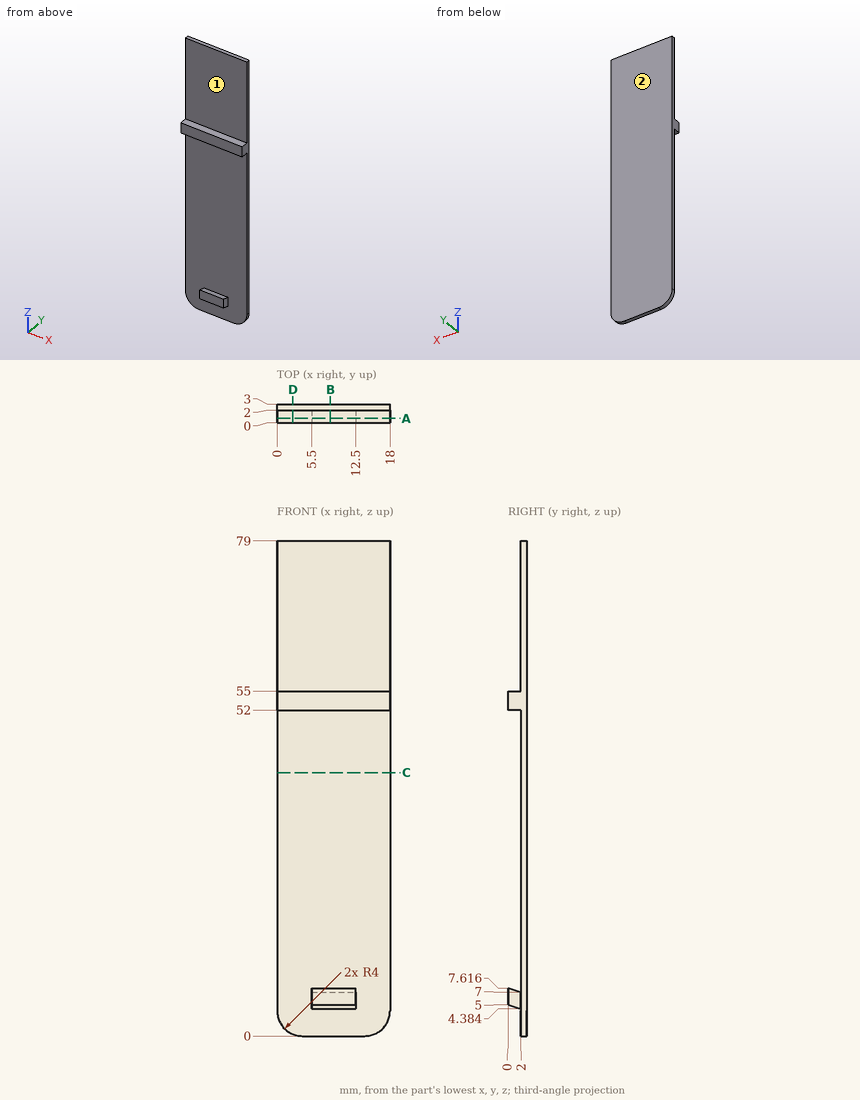
Part print with two shaded views. Sizes in mm from the minimum x, y, z corner. A direction names the side the tool comes from. Round coordinates to 2 decimals unless told otherwise and drop trailing zeros. Order: outer loops, then holes, each group sorted by start corner. A loop starts at its lowest first (then second) coordinate and runs counter-clockwise, first axis right, second up. Notation, with made-up numbers: (7.25, 71) - (50.25, 71) arc R18 ccw to (50.25, 103) - close; hole circle Ø7 at (33, -26). An arc over 180 degrees is marked (long way). Answer as CSV lines item,"result". Start each with the question number.
1. Saw through at B-B, the plane x = 8.5. Write the cut outline in (y, z).
2. Tool access for the marked faces 1 and 2: list every direction of +Z, -Z, +X, -X, +Y, -Y with a clear straight run to the whole face (end or side of a thin tool).
3. Saw through at C-C, the plane z = 42. Write the cut outline in (x, y).
4. Drill centre lines: L1, parallel to Y at x = 4.5, z = 13; L2, parallel to Z at x = 15.25, y = 1.1; L3, parallel to Z at x = 9, y = 1.2. Where is each one in solid material? Low to high. Write a range as [from, to].
5. Saw through at D-D, the plane x = 2.5. Write the cut outline in (y, z).
6. Saw through at A-A, the plane y = 0.7. Write the cut outline in (x, z).
7. Pin check, flat tips, straight feed: pin 1 (8 mm diameter, centred on x = 4, z = 64, fed in from -Y); pin 2 (0.6 mm diameter, centred on y = 1, z = 6, fed in from -X); pin 3 (1 mm diameter, centred on x = 2.5, y = 1, fed in from +Z). Stop position of each tip, or through.
Model answer:
1,outline,"(0, 5) - (2, 4.38) - (2, 0) - (3, 0) - (3, 79) - (2, 79) - (2, 55) - (0, 55) - (0, 52) - (2, 52) - (2, 7) - (0, 7.62) - close"
2,face 1,"+Z, +X, -X, -Y"
2,face 2,"+Z, -Z, +X, -X, +Y"
3,outline,"(0, 2) - (18, 2) - (18, 3) - (0, 3) - close"
4,L1,"y = [2, 3]"
4,L2,"z = [52, 55]"
4,L3,"z = [4.63, 7.25], [52, 55]"
5,outline,"(0, 52) - (2, 52) - (2, 0.29) - (3, 0.29) - (3, 79) - (2, 79) - (2, 55) - (0, 55) - close"
6,outline,"(0, 52) - (18, 52) - (18, 55) - (0, 55) - close; (5.5, 4.78) - (12.5, 4.78) - (12.5, 7.4) - (5.5, 7.4) - close"
7,pin 1,"stops at y = 2"
7,pin 2,"stops at x = 5.5"
7,pin 3,"stops at z = 55"
